The model under review builds one solid part; all positions refer to its coordinate system, in mm. Face numbers are marked on the shaded views. Round coordinates to 2 decimals unless told otherwise and drop trailing zeros. Order: outer loops, then holes, each group sorted by start corner. A loop starts at its lowest first (then second) coordinate and runs counter-clockwise, first axis right, second up. Notation, with made-up numbers: (27.5, 8) -> (34.5, 8) arc R27 ccw to (34.5, 35) -> close; hole circle Ø2 at (12, -0.5). An arc over 180 degrees is marked (long way). Return JSON: item names as keys, results as strings. Group by question number.
from build123d import *

# Parameters (mm, degrees)
SKETCH1_W           = 25
SKETCH1_H           = 30
SKETCH1_R           = 1.5
BOSS_EXTRUDE1_DEPTH = 3
SKETCH2_R           = 1.5
SKETCH2_R_2         = 2.5
SKETCH2_W           = 5
SKETCH2_H           = 6
CUT_EXTRUDE1_DEPTH  = 40.166312055
FILLET2_R           = 1


with BuildPart() as part:
    # Sketch1 → Boss-Extrude1 (new body)
    with BuildSketch(Plane(origin=(0, 0, 0), x_dir=(1, 0, 0), z_dir=(0, 1, 0))):
        with Locations((12.5, -15)):
            Rectangle(SKETCH1_W, SKETCH1_H)
        with Locations(Location((3, -20, 0), (0, 0, 270))):
            Circle(SKETCH1_R, mode=Mode.SUBTRACT)
        with Locations(Location((22, -20, 0), (0, 0, 270))):
            Circle(SKETCH1_R, mode=Mode.SUBTRACT)
        with Locations(Location((22, -3.18, 0), (0, 0, 270))):
            Circle(SKETCH1_R, mode=Mode.SUBTRACT)
        with Locations(Location((3, -3.18, 0), (0, 0, 270))):
            Circle(SKETCH1_R, mode=Mode.SUBTRACT)
    extrude(amount=BOSS_EXTRUDE1_DEPTH)

    # Sketch2 → Cut-Extrude1 (cut, through all)
    with BuildSketch(Plane(origin=(0, 3, 0), x_dir=(1, 0, 0), z_dir=(0, 1, 0))):
        with Locations(Location((12.5, -9.5, 0), (0, 0, 270))):
            Circle(SKETCH2_R)
        with Locations(Location((12.5, -17.5, 0), (0, 0, 270))):
            Circle(SKETCH2_R_2)
        with Locations((12.5, -3)):
            Rectangle(SKETCH2_W, SKETCH2_H)
    extrude(amount=-CUT_EXTRUDE1_DEPTH, mode=Mode.SUBTRACT)

    # Fillet2
    fillet2_edges = [part.edges().sort_by_distance(p)[0] for p in [
        (10, 1.5, 0),
        (15, 1.5, 0),
        (0, 1.5, 0),
        (25, 1.5, 0),
        (25, 1.5, 30),
        (0, 1.5, 30),
    ]]
    fillet(fillet2_edges, radius=FILLET2_R)


solid = part.part
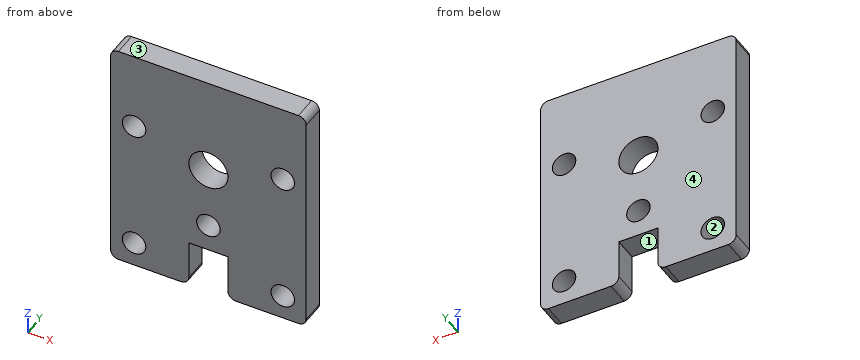
Item 1: Consider section A-A on z = 17.5. State the section outline as (x, y) points, plus the area to 3 significant figures.
Item 2: Wall thickness on line 1 along X through (y, z) = (1.9, 3.18); line 2 along X through (y, z) = (2.75, 21.25); line 3 along Z through (x, y) = (3.5, 0.4): over which ranges is each line inside the solid? List them lowest first.
Item 3: Consider section B-B on z = 3.18. State the section outline as (x, y) points, plus the area to 3 significant figures.
Item 4: The part is to be moulded in two halves that separate along Z. For the marked faces 1, 2, 3 and 4, say which applies: +Z half, -Z half, draft (parallel to the pull), parting line (faces both ways), or undercut.
Item 5: Consider section D-D on y = 2.5. State the section outline as (x, z) points, plus the area to 3 significant figures.
Item 6: Consider section C-C on x = 12.5. State the section outline as (y, z) points, plus the area to 3 significant figures.
Values:
{
 "1": {"outline": "(0, 0) -> (10, 0) -> (10, 3) -> (0, 3) -> close; (15, 0) -> (25, 0) -> (25, 3) -> (15, 3) -> close", "area": "60.0 mm^2"},
 "2": {"line 1": "0 to 1.5, 4.5 to 10, 15 to 20.5, 23.5 to 25", "line 2": "0 to 2.17, 3.83 to 21.17, 22.83 to 25", "line 3": "0 to 1.77, 4.59 to 18.59, 21.41 to 30"},
 "3": {"outline": "(0, 0) -> (1.5, 0) -> (1.5, 3) -> (0, 3) -> close; (4.5, 0) -> (10, 0) -> (10, 3) -> (4.5, 3) -> close; (15, 0) -> (20.5, 0) -> (20.5, 3) -> (15, 3) -> close; (23.5, 0) -> (25, 0) -> (25, 3) -> (23.5, 3) -> close", "area": "42.0 mm^2"},
 "4": {"face 1": "-Z half", "face 2": "undercut", "face 3": "+Z half", "face 4": "draft"},
 "5": {"outline": "(0, 1) arc R1 ccw to (1, 0) -> (9, 0) arc R1 ccw to (10, 1) -> (10, 6) -> (15, 6) -> (15, 1) arc R1 ccw to (16, 0) -> (24, 0) arc R1 ccw to (25, 1) -> (25, 29) arc R1 ccw to (24, 30) -> (1, 30) arc R1 ccw to (0, 29) -> close; hole circle Ø3 at (3, 3.18); hole circle Ø3 at (3, 20); hole circle Ø5 at (12.5, 17.5); hole circle Ø3 at (12.5, 9.5); hole circle Ø3 at (22, 3.18); hole circle Ø3 at (22, 20)", "area": "664 mm^2"},
 "6": {"outline": "(0, 6) -> (3, 6) -> (3, 8) -> (0, 8) -> close; (0, 11) -> (3, 11) -> (3, 15) -> (0, 15) -> close; (0, 20) -> (3, 20) -> (3, 30) -> (0, 30) -> close", "area": "48.0 mm^2"}
}
